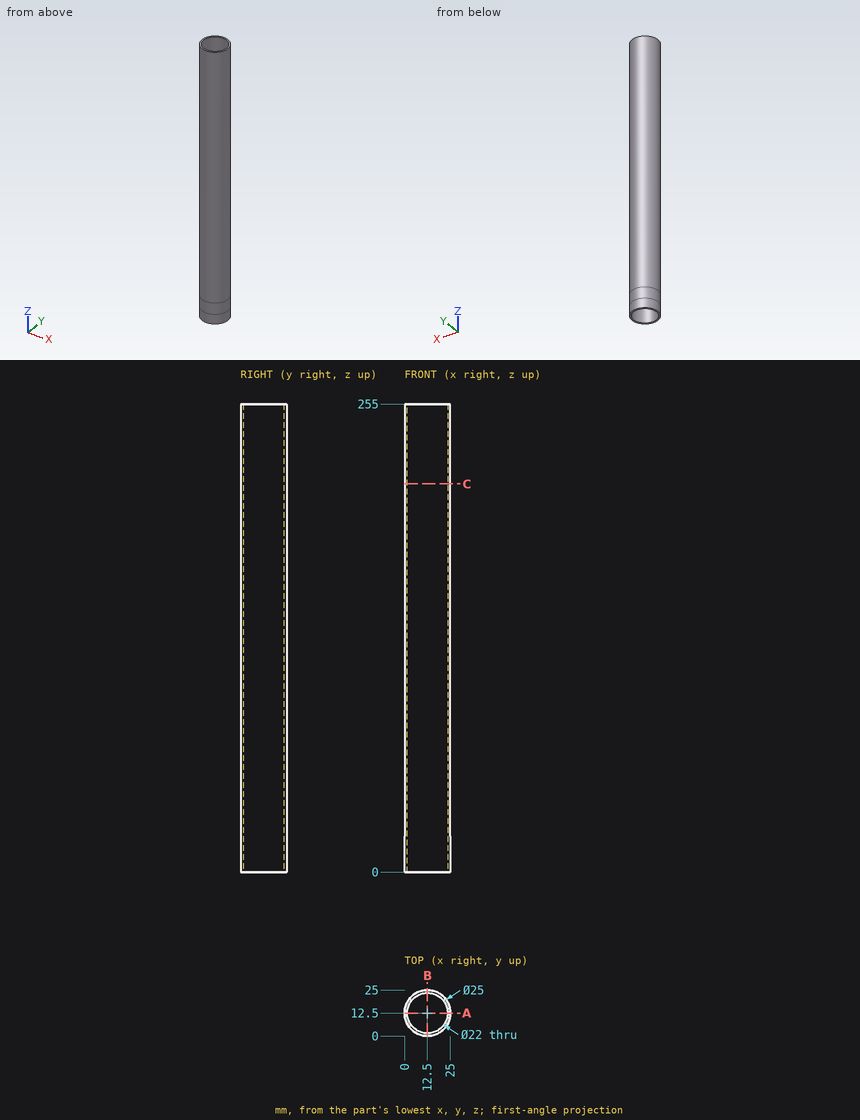
Verification items for this drawing (mm, ordinates from the low corner). Coordinates: 2 decimals unless noted, no trailing zeros. Order: outer loops, then holes, each group sorted by start corner. A loop starts at its lowest first (then second) coordinate and runs counter-clockwise, first axis right, second up. Notation, with made-up numbers: (-12.75, 43.25) -> (35.25, 43.25) arc R18 cw to (35.25, 51.25) -> close; hole circle Ø2 at (37.25, 23). An arc over 180 degrees is marked (long way). Answer as CSV lines item,"result". Start each with the question number.
1) Cross-section at A-A, the plane y = 12.5. Record the boundary of the cut face in (x, z), then the cut area to 3 significant figures.
2) Cross-section at C-C, the plane z = 211.5. Record the boundary of the cut face in (x, y).
3) Gauge pin test, flat ends, axial feed: pin 1 Ø10 at (x, z) = (19.5, 204) entering from -Y; pin 2 Ø4 at (y, z) = (15.5, 70.5) entering from +X; pin 3 Ø2 at (x, z) = (11, 215) entering from -Y; pin 4 Ø12 at (x, z) = (16.5, 105.5) entering from +Y. Record the tip position at first contact, or that the pin passes through.
4) Material ranges on L1, parallel to Y at x = 12.5, z = 80; L2, parallel to X at y = 22, z = 121.5; L3, parallel to Y at x = 22.5, z = 187, recorded low to high. Write a range as [from, to].
Conclusion:
1,outline,"(0, 0) -> (1.5, 0) -> (1.5, 255) -> (0, 255) -> close; (23.5, 0) -> (25, 0) -> (25, 255) -> (23.5, 255) -> close"
1,area,"765 mm²"
2,outline,"circle Ø25 at (12.5, 12.5); hole circle Ø22 at (12.5, 12.5)"
3,pin 1,"stops at y = 0.16"
3,pin 2,"stops at x = 24.96"
3,pin 3,"stops at y = 0.01"
3,pin 4,"stops at y = 25"
4,L1,"y = [0, 1.5], [23.5, 25]"
4,L2,"x = [4.38, 6.95], [18.05, 20.62]"
4,L3,"y = [5, 7.92], [17.08, 20]"
